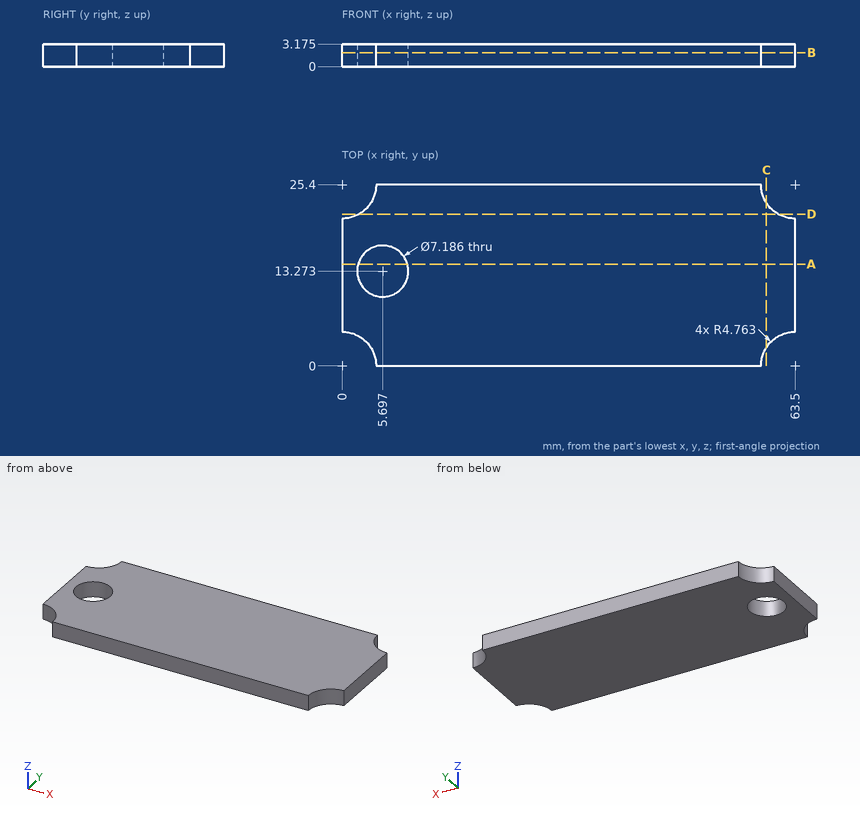
Verification items for this drawing (mm, ordinates from the low corner). Coordinates: 2 decimals unless noted, no trailing zeros. Loops run counter-clockwise (first coordinate to the right, second up) from the corner with the lowest first, then second, coordinate; pieces in that order, holes last.
Item 1: Sectioned sample at B-B, the plane z = 1.95. Record the boundary of the cut face in (x, y) (1 decimal), then the cut area to 3 significant figures.
Item 2: Sectioned sample at A-A, the plane y = 14.25. Record the boundary of the cut face in (x, z) (1 decimal), then the cut area to 3 significant figures.
Item 3: Thickness scan on line 1 (X direction, y = 15, z = 2.45) (1 decimal); line 2 (X direction, y = 11, z = 2.9) (1 decimal); line 3 (X direction, y = 22.5, z = 1.55). Record the ranges inside material, lowest first.
Item 4: Sectioned sample at C-C, the plane x = 59.5. Record the boundary of the cut face in (y, z) (1 decimal).
Item 5: Go/stop test with a flat-tipped pin: pin 1 Ø1.5 at (x, y) = (36.5, 4.5) entering from -Z. Record where the tip stops, or that it passes through.
Item 6: Sectioned sample at D-D, the plane y = 21.25. Record the boundary of the cut face in (x, z) (1 decimal).
Check result:
1. outline: (0, 4.8) arc R4.8 cw to (4.8, 0) - (58.7, 0) arc R4.8 cw to (63.5, 4.8) - (63.5, 20.6) arc R4.8 cw to (58.7, 25.4) - (4.8, 25.4) arc R4.8 cw to (0, 20.6) - close; hole circle Ø7.2 at (5.7, 13.3)
1. area: 1,500 mm2
2. outline: (0, 0) - (2.2, 0) - (2.2, 3.2) - (0, 3.2) - close; (9.2, 0) - (63.5, 0) - (63.5, 3.2) - (9.2, 3.2) - close
2. area: 180 mm2
3. line 1: x = 0 to 2.5, 8.8 to 63.5
3. line 2: x = 0 to 2.9, 8.5 to 63.5
3. line 3: x = 3.78 to 59.72
4. outline: (2.6, 0) - (22.8, 0) - (22.8, 3.2) - (2.6, 3.2) - close
5. pin 1: stops at z = 0
6. outline: (2.3, 0) - (61.2, 0) - (61.2, 3.2) - (2.3, 3.2) - close
